from build123d import *

# Parameters (mm, degrees)
F0_W     = 474.8173340189
F0_H     = 406.4
F1_DEPTH = 25.4
F3_DEPTH = 25.4
F4_W     = 317.5059556961
F4_H     = 358.9637875557
F5_DEPTH = 25.4
F7_DEPTH = 25.4


with BuildPart() as f1:
    # F0 (on Front) → F1 (new body)
    with BuildSketch(Plane.XZ):
        with Locations((-2.3857876658, 9.4393342733)):
            Rectangle(F0_W, F0_H)
    extrude(amount=F1_DEPTH)

    # F2 (on face) → F3 (cut)
    with BuildSketch(Plane.XZ.offset(25.4)):
        with BuildLine():
            ThreePointArc((-239.7944546753, -5.535e-07), (-205.0373357652, 124.3425568152), (-110.841752119, 212.6393342733))
            Line((-110.841752119, 212.6393342733), (-239.7944546753, 212.6393342733))
            Line((-239.7944546753, 212.6393342733), (-239.7944546753, -5.535e-07))
        make_face()
        with BuildLine():
            Line((-239.7944546753, -193.7606657267), (-141.273440215, -193.7606657267))
            ThreePointArc((-141.273440215, -193.7606657267), (-213.7498163066, -108.6848495509), (-239.7944546753, -5.535e-07))
            Line((-239.7944546753, -5.535e-07), (-239.7944546753, -193.7606657267))
        make_face()
    extrude(amount=-F3_DEPTH, mode=Mode.SUBTRACT)

    # F4 (on face) → F5 (cut)
    with BuildSketch(Plane.XZ.offset(25.4)):
        with Locations((53.7397265434, 5.900233984)):
            Rectangle(F4_W, F4_H)
    extrude(amount=-F5_DEPTH, mode=Mode.SUBTRACT)

    # F6 (on face) → F7 (cut)
    with BuildSketch(Plane.XZ.offset(25.4)):
        with BuildLine():
            Line((-105.0132513046, -173.5816597939), (-105.0132513046, 185.3821277618))
            ThreePointArc((-105.0132513046, 185.3821277618), (-214.776070383, 5.900233984), (-105.0132513046, -173.5816597939))
        make_face()
    extrude(amount=-F7_DEPTH, mode=Mode.SUBTRACT)


solid = f1.part
Source: CAD feature listing. Evaluate the final solid. Frame: model axes, mm. A direction names the side the tool comes from. Round coordinates to 2 decimals unless told otherwise and drop trailing zeros. Loops run counter-clockwise (first coordinate to the right, second up) from the corner with the lowest first, then second, coordinate; pieces in that order, holes last. Notation, with made-up numbers: (36.5, 43) - (84.5, 43) arc R27 ccw to (84.5, 66) - close; hole circle Ø8 at (75, 56). An arc over 180 degrees is marked (long way). Write item = value, one per line. Start each with the question number.
(1) Pull-direction query (Z, two-part tool) for faces 1 (the face through (60, -13, 212.639)), 2 (the face through (235.023, -13, 7)), 3 (the face through (-214.752, -12.878, 8.999)); classes: +Z half, -Z half, draft (parallel to the pull), parting line (faces both ways), or undercut.
(2) Section query A-A, the plane x = 177.5. Output: boundary loops of the cut face in (y, z).
(3) Pin query (flat end, axial travel): pin 1 (12 mm diameter, centred on x = -165.5, y = -11.5, fed in from -Z). Return the tip coordinate at first contact, or that it passes through.
(4) Ray query, line 1 along Z through (x, y) = (160.5, -20.75); line 2 along X through (y, z) = (-10.25, -10); line 3 along X through (y, z) = (-7.75, 68.5). Return the intervals inside material, ascending. Write a range as from..to.
(5) Set-up query: faces 4 (the face through (212.493, -13, 3)), 5 (the face through (44, -13, -193.761)). Return all of +Z, -Z, +X, -X, +Y, -Y with unobstructed straight access to the full face (end or side cutting, diameter ignored); none if empty.
(6) Section query C-C, the plane z = 41. Output: boundary loops of the cut face in (x, y), plus the area to 3 significant figures.
(7) Section query B-B, the plane y = -6.75. Output: boundary loops of the cut face in (x, z).
Conclusion:
q1.face_1 = +Z half
q1.face_2 = draft
q1.face_3 = undercut
q2.outline = (-25.4, -193.76) - (0, -193.76) - (0, -173.58) - (-25.4, -173.58) - close; (-25.4, 185.38) - (0, 185.38) - (0, 212.64) - (-25.4, 212.64) - close
q3.pin_1 = -179.06
q4.line_1 = -193.76..-173.58, 185.38..212.64
q4.line_2 = -239.59..-214.15, 212.49..235.02
q4.line_3 = -229.8..-204.81, 212.49..235.02
q5.face_4 = +Y, -Y
q5.face_5 = -Z, +X, -X, +Y, -Y
q6.outline = (-236.26, -25.4) - (-211.7, -25.4) - (-211.7, 0) - (-236.26, 0) - close; (212.49, -25.4) - (235.02, -25.4) - (235.02, 0) - (212.49, 0) - close
q6.area = 1,200 mm2
q7.outline = (-141.27, -193.76) - (235.02, -193.76) - (235.02, 212.64) - (-110.84, 212.64) arc R239.79 ccw to start; hole (-105.01, -173.58) - (212.49, -173.58) - (212.49, 185.38) - (-105.01, 185.38) arc R201.62 ccw to start
